Geometry check sheet. Reference: the model listing, model coordinates, mm. Face numbers are marked on the shaded views. Round coordinates to 2 decimals unless told otherwise and drop trailing zeros. Write each loop counter-clockwise with the first axis right and the second up, starting at its lowest first coordinate (ties: lowest second). Pieces come first, ordered by that corner, then holes. Notation, with made-up numbers: M 54,57.5 L 73,57.5 A14 cw 73,74.5 Z; hole C -39.75,1 d4. An arc over 180 degrees is marked long. Put each result on its own line as item: value. Start each with the question number.
(1) Mould release check, pull along X, two halves, no side actions. Record for the marked faces 1 and 2: pulls with the +X half, pulls with the -X half, needs draft (parallel to the pull), parting line crosses it, or undercut.
(2) Gauge pin test, flat ends, axial feed: pin 1 (4 mm diameter, centred on x = -13.5, z = 20.5, fed in from -Y); pin 2 (6 mm diameter, centred on x = -16.42, y = -4.4, fed in from +Z); pin 3 (3 mm diameter, centred on y = 7.5, z = 22, fed in from +X); pin 4 (5 mm diameter, centred on x = -16.42, z = 20, fed in from +Y). Record the tip position at first contact, or that the pin passes through.
(3) Section check A-A on x = 0. Record the cut outline in (y, z).
(4) Section check D-D on y = 10.5. Record the cut outline in (x, z), then the cut area to 3 significant figures.
(5) Section check C-C on z = 21. Record the cut outline in (x, y).
(6) Section check B-B on y = -5.5. Record the cut outline in (x, z).
(7) Material ranges on probe 1 along X at (y, z) = (-1.5, 22.5); probe 2 along Y at (x, z) = (-16, 13); probe 3 along Y at (x, z) = (0.5, 31), recorded low to high.
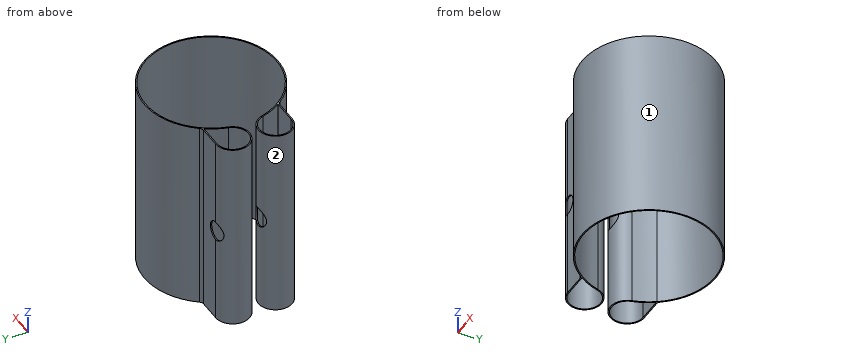
from build123d import *

# Parameters (mm, degrees)
F1_DEPTH = 40
F2_R     = 1
F3_R     = 2
F4_DEPTH = 25


with BuildPart() as f1:
    # F0 (on Top) → F1 (new body)
    with BuildSketch(Plane.XY):
        with BuildLine():
            ThreePointArc((-11.123339, 7.649924), (13.304653, -2.288275), (-13.039999, -3.494057))
            ThreePointArc((-13.039999, -3.494057), (-19.197476, -2.269259), (-16.420739, -7.899924))
            Line((-16.420739, -7.899924), (-11.254053, -7.899924))
            ThreePointArc((-11.254053, -7.899924), (13.75, 0), (-11.254053, 7.899924))
            ThreePointArc((-11.254053, 7.899924), (-11.340446, 7.775396), (-11.425461, 7.649924))
            Line((-11.425461, 7.649924), (-11.123339, 7.649924))
        make_face()
        with BuildLine():
            ThreePointArc((-16.420739, -7.649924), (-18.999137, -2.421449), (-13.28148, -3.558762))
            ThreePointArc((-13.28148, -3.558762), (-12.521687, -5.680657), (-11.425461, -7.649924))
            Line((-11.425461, -7.649924), (-15.121701, -7.649924))
            Line((-15.121701, -7.649924), (-16.420739, -7.649924))
        make_face(mode=Mode.SUBTRACT)
        with BuildLine():
            ThreePointArc((-13.039999, 3.494057), (-12.259059, 5.653802), (-11.123339, 7.649924))
            Line((-11.123339, 7.649924), (-11.425461, 7.649924))
            ThreePointArc((-11.425461, 7.649924), (-11.340446, 7.775396), (-11.254053, 7.899924))
            Line((-11.254053, 7.899924), (-16.420739, 7.899924))
            ThreePointArc((-16.420739, 7.899924), (-19.197476, 2.269259), (-13.039999, 3.494057))
        make_face()
        with BuildLine():
            Line((-15.121701, 7.649924), (-11.425461, 7.649924))
            ThreePointArc((-11.425461, 7.649924), (-12.521687, 5.680657), (-13.28148, 3.558762))
            ThreePointArc((-13.28148, 3.558762), (-18.999137, 2.421449), (-16.420739, 7.649924))
            Line((-16.420739, 7.649924), (-15.121701, 7.649924))
        make_face(mode=Mode.SUBTRACT)
    extrude(amount=F1_DEPTH)

    # F2
    f2_edges = [f1.edges().sort_by_distance(p)[0] for p in [
        (-11.254053, 7.899924, 20),
        (-11.254053, -7.899924, 20),
    ]]
    fillet(f2_edges, radius=F2_R)

    # F3 (on face) → F4 (cut)
    with BuildSketch(Plane(origin=(0, 7.899924, 0), x_dir=(-1, 0, 0), z_dir=(0, 1, 0))):
        with Locations((16.420739, 20)):
            Circle(F3_R)
    extrude(amount=-F4_DEPTH, mode=Mode.SUBTRACT)


solid = f1.part
Answers follow:
1. face 1: parting line crosses it
1. face 2: undercut
2. pin 1: stops at y = -7.93
2. pin 2: passes through
2. pin 3: stops at x = 12.37
2. pin 4: stops at y = 7.9
3. outline: M -13.75,0 L -13.5,0 L -13.5,40 L -13.75,40 Z; M 13.5,0 L 13.75,0 L 13.75,40 L 13.5,40 Z
4. outline: M -8.88,0 L -8.49,0 L -8.49,40 L -8.88,40 Z; M 8.49,0 L 8.88,0 L 8.88,40 L 8.49,40 Z
4. area: 31.4 mm^2
5. outline: M -18.15,-7.44 L -18.15,-7.15 A3.25 cw -18.15,-1.65 L -18.15,-1.36 A3.5 ccw Z; M -18.15,1.36 L -18.15,1.65 A3.25 cw -18.15,7.15 L -18.15,7.44 A3.5 ccw Z; M -14.69,-7.9 L -11.76,-7.9 A1 cw -10.96,-8.3 A13.75 ccw long -10.96,8.3 A1 cw -11.76,7.9 L -14.69,7.9 L -14.69,7.65 L -11.43,7.65 A13.75 ccw -13.28,3.56 A3.25 cw -14.69,1.65 L -14.69,1.36 A3.5 ccw -13.04,3.49 A13.5 cw -11.12,7.65 A13.5 cw long -13.04,-3.49 A3.5 ccw -14.69,-1.36 L -14.69,-1.65 A3.25 cw -13.28,-3.56 A13.75 ccw -11.43,-7.65 L -14.69,-7.65 Z
6. outline: M -19.74,0 L -19.48,0 L -19.48,40 L -19.74,40 Z; M -12.6,0 L -12.33,0 L -12.33,40 L -12.6,40 Z; M 12.33,0 L 12.6,0 L 12.6,40 L 12.33,40 Z
7. probe 1: x = -18.38 to -17.89, -14.95 to -14.46, 13.42 to 13.67
7. probe 2: y = -7.9 to -7.65, -1.18 to -0.93, 0.93 to 1.18, 7.65 to 7.9
7. probe 3: y = -13.74 to -13.49, 13.49 to 13.74
